from build123d import *

# Parameters (mm, degrees)
BASPROSKE_W             = 6
BASPROSKE_H             = 12.75
TOOTHCUT_DEPTH          = 20.003289189
TEETHCUTS_COUNT         = 15
TEETHCUTS_ANGLE         = 336
BORSKE_R                = 3
BORE_DEPTH              = 50.0000508
BOSS_EXTRUDE2_START     = 6
SKETCH1_R               = 6
SKETCH1_R_2             = 3
BOSS_EXTRUDE2_DEPTH     = 6
CUT_EXTRUDE1_START      = -6.0000001
CUT_EXTRUDE1_OUTLINE_W  = 6
CUT_EXTRUDE1_OUTLINE_H  = 2
CUT_EXTRUDE1_DEPTH      = 3.171572975
SKETCH3_W               = 6
SKETCH3_H               = 7.395975174
BOSS_EXTRUDE3_DEPTH     = 1.5
BOSS_EXTRUDE4_DEPTH     = 1.5
CUT_EXTRUDE2_DEPTH      = 23.109303185
CUT_EXTRUDE2_DEPTH_BACK = 23.109303185
SKETCH6_R               = 1.5
CUT_EXTRUDE3_DEPTH      = 24.197646745


# Read off the part's stored shape, not the designer's step: Cut-Extrude1
with BuildPart() as part:
    # BasProSke → Base-Revolve (revolve)
    with BuildSketch(Plane(origin=(0, 0, 0), x_dir=(1, 0, 0), z_dir=(0, 1, 0)), mode=Mode.PRIVATE) as base_revolve_sk:
        with Locations((3, 6.375)):
            Rectangle(BASPROSKE_W, BASPROSKE_H)
    revolve(base_revolve_sk.sketch.rotate(Axis((-10, 0, 0), (1, 0, 0)), 180), axis=Axis((-10, 0, 0), (1, 0, 0)))

    # TooCutSke → ToothCut (cut, through all)
    with BuildSketch(Plane(origin=(0, 0, 0), x_dir=(0, 0, -1), z_dir=(1, 0, 0))):
        with BuildLine():
            ThreePointArc((0.791546546, 9.340520867), (0, 9.374), (-0.791546546, 9.340520867))
            ThreePointArc((-0.791546546, 9.340520867), (-1.235070734, 11.110218102), (-2.344732916, 12.558386549))
            ThreePointArc((-2.344732916, 12.558386549), (0, 12.7754), (2.344732916, 12.558386549))
            ThreePointArc((2.344732916, 12.558386549), (1.235070734, 11.110218102), (0.791546546, 9.340520867))
        make_face()
    toothcut = extrude(amount=TOOTHCUT_DEPTH, mode=Mode.SUBTRACT)

    # TeethCuts: ToothCut ×15 about axis
    teethcuts_axis = Axis((-10, 0, 0), (1, 0, 0))
    for i in range(1, TEETHCUTS_COUNT):
        add(toothcut.rotate(teethcuts_axis, i * TEETHCUTS_ANGLE / (TEETHCUTS_COUNT - 1)), mode=Mode.SUBTRACT)

    # BorSke → Bore (cut, symmetric)
    with BuildSketch(Plane(origin=(0, 0, 0), x_dir=(0, 0, -1), z_dir=(1, 0, 0))):
        with Locations(Location((0, 0, 0), (0, 0, 180))):
            Circle(BORSKE_R)
    extrude(amount=BORE_DEPTH, both=True, mode=Mode.SUBTRACT)

    # Sketch1 → Boss-Extrude2 (add)
    with BuildSketch(Plane(origin=(6, 0, 0), x_dir=(0, 0, -1), z_dir=(1, 0, 0)).offset(BOSS_EXTRUDE2_START)):
        with Locations(Location((0, 0, 0), (0, 0, 180))):
            Circle(SKETCH1_R)
        Circle(SKETCH1_R_2, mode=Mode.SUBTRACT)
    extrude(amount=-BOSS_EXTRUDE2_DEPTH)

    # Cut-Extrude1 outline → Cut-Extrude1 (cut)
    with BuildSketch(Plane.XY.offset(CUT_EXTRUDE1_START)):
        with Locations((9, 0)):
            Rectangle(CUT_EXTRUDE1_OUTLINE_W, CUT_EXTRUDE1_OUTLINE_H)
    extrude(amount=CUT_EXTRUDE1_DEPTH, mode=Mode.SUBTRACT)

    # Sketch3 → Boss-Extrude3 (add)
    with BuildSketch(Plane(origin=(0, -1, 0), x_dir=(1, 0, 0), z_dir=(0, 1, 0))):
        with Locations((9, 6.526414712)):
            Rectangle(SKETCH3_W, SKETCH3_H)
    extrude(amount=-BOSS_EXTRUDE3_DEPTH)

    # Sketch5 → Boss-Extrude4 (add)
    with BuildSketch(Plane.XZ.offset(-1)):
        Polygon((6, -10.224402299), (6, -9.320508355), (6, -2.828427125), (12, -2.828427125), (12, -10.224402299), align=None)
    extrude(amount=-BOSS_EXTRUDE4_DEPTH)

    # Sketch6 → Cut-Extrude2 (cut, two sides: drawn at the far end of the back side and taken through both)
    with BuildSketch(Plane(origin=(0, -1, 0), x_dir=(1, 0, 0), z_dir=(0, 1, 0)).offset(-CUT_EXTRUDE2_DEPTH_BACK)):
        with Locations(Location((9, 6.526414712, 0), (0, 0, 270))):
            Circle(SKETCH6_R)
    extrude(amount=CUT_EXTRUDE2_DEPTH + CUT_EXTRUDE2_DEPTH_BACK, mode=Mode.SUBTRACT)

    # Sketch7 → Cut-Extrude3 (cut, through all)
    with BuildSketch(Plane(origin=(0, 2.5, 0), x_dir=(1, 0, 0), z_dir=(0, 1, 0))):
        with BuildLine():
            ThreePointArc((6.901724288, 4.382297403), (9, 3.526414712), (11.098275712, 4.382297403))
            ThreePointArc((11.098275712, 4.382297403), (9, 9.526414712), (6.901724288, 4.382297403))
        make_face()
    extrude(amount=CUT_EXTRUDE3_DEPTH, mode=Mode.SUBTRACT)


solid = part.part
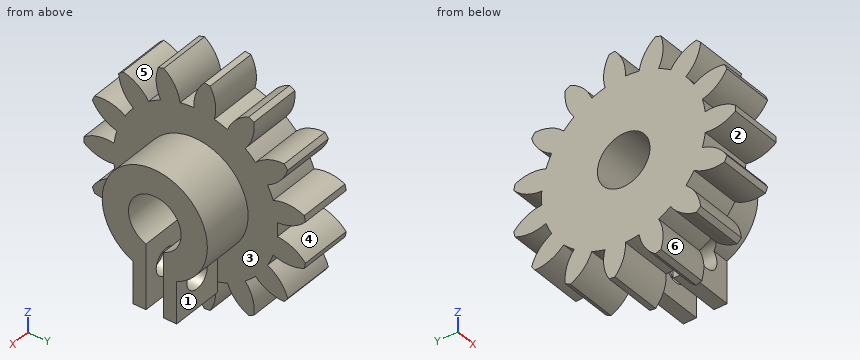
Model file for the job. Use its own axes, mm. Face numbers are marked on the shaded views. A direction names the side the tool comes from. Coordinates: 2 decimals unless noted, no trailing zeros. Order: outer loops, then holes, each group sorted by start corner. A loop starts at its lowest first (then second) coordinate and runs counter-clockwise, first axis right, second up. Notation, with made-up numbers: M 6,-16.75 L 30,-16.75 A27 ccw 30,9.25 Z; hole C -13,79.25 d10. An arc over 180 degrees is marked long. Return JSON: item names as keys, results as strings.
1. Saw through at B-B (x = 9). Give the cut face in (y, z), and give its area (3 significant figures).
Ans:
{"outline": "M -3.28,-5.03 L -1,-5.03 L -1,-2.83 A3 cw long 1,-2.83 L 1,-5.03 L 2.5,-5.03 L 2.5,-3.53 L 4.85,-3.53 A6 ccw long Z; M -2.5,-10.22 L -1,-10.22 L -1,-8.03 L -2.5,-8.03 Z; M 1,-10.22 L 2.5,-10.22 L 2.5,-8.03 L 1,-8.03 Z", "area": "80.4 mm^2"}
2. Flat gauge pins, fed straight in: pin 1 (6.5 mm diameter, centred on x = 7.5, z = -7.5, fed in from -Y); pin 2 (5 mm diameter, centred on x = 3.5, z = 5, fed in from +Y); pin 3 (1.8 mm diameter, centred on x = 8, z = -6, fed in from +Y). Where does each tip first touch, or does it go through?
Ans:
{"pin 1": "y = -11.78", "pin 2": "y = 12.5", "pin 3": "y = 2.5"}
3. Saw through at C-C (z = 10.5). Give the cut face in (x, y), and give its area (3 significant figures).
Ans:
{"outline": "M 0,-4.5 L 6,-4.5 L 6,-2.16 L 0,-2.16 Z; M 0,-0.12 L 6,-0.12 L 6,2.3 L 0,2.3 Z; M 0,4.94 L 6,4.94 L 6,6.69 L 0,6.69 Z", "area": "39.0 mm^2"}
4. Drill centre lines: probe 1 along Z at (x, y) = (9, 1.4); probe 2 along Y at (x, z) = (3.75, -10); probe 3 along Z at (x, y) = (9, 1.6). Where is each one in solid material? Low to high.
Ans:
{"probe 1": "-10.22 to -8.03, -5.03 to -2.65, 2.65 to 5.83", "probe 2": "-4.46 to -1.96, -0.19 to 2.29, 4.44 to 6.68", "probe 3": "-10.22 to -8.03, -5.03 to -2.54, 2.54 to 5.78"}
5. Pull direction X, two halves, no side cores. Call the marked faces 1, 2 and 3: +X half, -X half, draft (parallel to the pull), parting line (faces both ways), or undercut.
Ans:
{"face 1": "undercut", "face 2": "draft", "face 3": "+X half"}
6. Saw through at A-A (z = 0). Give the cut face in (x, y).
Ans:
{"outline": "M 0,-12.75 L 6,-12.75 L 6,-6 L 12,-6 L 12,-3 L 0,-3 Z; M 0,3 L 12,3 L 12,6 L 6,6 L 6,9.37 L 0,9.37 Z"}
7. Saw through at D-D (y = 5.25). Give the cut face in (x, z), and give its area (3 significant figures).
Ans:
{"outline": "M 0,-10.74 L 6,-10.74 L 6,-2.9 L 12,-2.9 L 12,2.9 L 6,2.9 L 6,10.74 L 0,10.74 Z", "area": "164 mm^2"}
8. Tool access for the marked faces 4, 5 and 6: list every direction of +Z, -Z, +X, -X, +Y, -Y with a clear straight run to the whole face (end or side of a thin tool).
Ans:
{"face 4": "+X, -X, +Y", "face 5": "+Z, +X, -X", "face 6": "+X, -X"}
